```python
from build123d import *

# Parameters (mm, degrees)
SKETCH1_W           = 127
SKETCH1_H           = 266.7
BOSS_EXTRUDE1_DEPTH = 25.4
SHELL1_T            = -3.175
SKETCH2_R           = 9.525
SKETCH2_R_2         = 3.175
BOSS_EXTRUDE2_DEPTH = 3.175
BOSS_EXTRUDE3_DEPTH = 38.1


with BuildPart() as part:
    # Sketch1 → Boss-Extrude1 (new, symmetric)
    with BuildSketch(Plane.XY):
        Rectangle(SKETCH1_W, SKETCH1_H)
    extrude(amount=BOSS_EXTRUDE1_DEPTH, both=True)

    # Shell1
    shell1_openings = [part.faces().sort_by_distance(p)[0] for p in [
        (0, 0, 25.4),
    ]]
    offset(amount=SHELL1_T, openings=shell1_openings, kind=Kind.INTERSECTION)

    # Sketch2 → Boss-Extrude2 (add)
    with BuildSketch(Plane.ZY.offset(63.5)):
        with BuildLine():
            Line((50.8, 130.175), (25.4, 130.175))
            Line((25.4, 130.175), (25.4, 53.975))
            Line((25.4, 53.975), (44.45, 53.975))
            ThreePointArc((44.45, 53.975), (55.181439518, 59.883372369), (55.927786008, 72.11103057))
            ThreePointArc((55.927786008, 72.11103057), (54.690903616, 84.99461885), (61.97223251, 95.695038213))
            ThreePointArc((61.97223251, 95.695038213), (68.922407015, 116.99704087), (50.8, 130.175))
        make_face()
        with Locations(Location((50.8, 111.125, 0), (0, 0, 270))):
            Circle(SKETCH2_R, mode=Mode.SUBTRACT)
        with Locations(Location((44.45, 66.675, 0), (0, 0, 270))):
            Circle(SKETCH2_R_2, mode=Mode.SUBTRACT)
    boss_extrude2 = extrude(amount=-BOSS_EXTRUDE2_DEPTH)

    # Sketch3 → Boss-Extrude3 (add)
    with BuildSketch(Plane(origin=(0, 133.35, 0), x_dir=(1, 0, 0), z_dir=(0, 1, 0))):
        with BuildLine():
            Line((63.5, -25.4), (-63.5, -25.4))
            Line((-63.5, -25.4), (-63.5, 38.1))
            Line((-63.5, 38.1), (25.4, 38.1))
            ThreePointArc((25.4, 38.1), (52.340768363, 26.940768363), (63.5, 0))
            Line((63.5, 0), (63.5, -25.4))
        make_face()
    extrude(amount=BOSS_EXTRUDE3_DEPTH)

    # Mirror1: Boss-Extrude2 across plane
    add(boss_extrude2.mirror(Plane.ZX))


solid = part.part
```
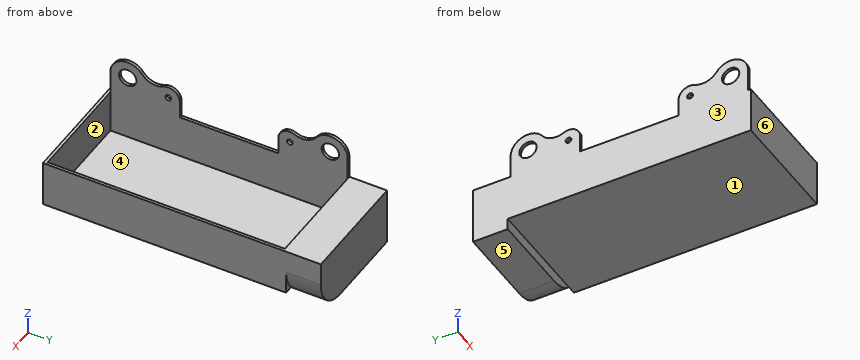
For this review, take the finished solid that the model builds, in its own axes (mm). Face numbers are marked on the shaded views. A direction names the side the tool comes from. Give positions to 0.01 mm unless a question says otherwise; leave off trailing zeros. Loops run counter-clockwise (first coordinate to the right, second up) from the corner with the lowest first, then second, coordinate; pieces in that order, holes last. Notation, with made-up numbers: M 21,-1 L 74,-1 A28 cw 74,29 Z; hole C 84.5,59 d7. An arc over 180 degrees is marked long. One line per item, written item: value. Start each with the question number.
Q1. Add section C-C (y = 139). Give the boundary of the cut face in (x, z).
Q2. For L1, parallel to X at y = -67, z = -5.5 (3 decimals); L2, parallel to Y at x = 24.5, z = -1.5 (3 decimals); L3, parallel to Z at x = 23.5, y = 33 (3 decimals), list the stretches that pass through material, from the lowest coordinate up.
Q3. Add section B-B (x = -51.5). Give the boundary of the cut face in (y, z) (3 decimals), and give its area (3 significant figures).
Q4. Add section A-A (y = 38). Give the boundary of the cut face in (x, z) (3 decimals), and give its area (3 significant figures).
Q5. Add section D-D (x = 39.5). Give the boundary of the cut face in (y, z) (3 decimals).
Q6. Draft analysis for pull direction Y (two halves, no side actions). For the marked faces 4, 5 and 6, state which applies: released by +Y, released by -Y, zero draft, split by the parting line, or undercut.
Q7. Machinability: for the marked faces 1, 2 and 3, which of the approach directions +Z, -Z, +X, -X, +Y, -Y give a long, thin tool a straight path to every point of the face, cutting with its end or side? Answer none if there is none.
Q8. Clearance check with flat-ended pins moving along their axes: pin 1 Ø2 at (x, y) = (27, 69) entering from +Z (3 decimals); pin 2 Ø8 at (x, y) = (22.5, 102) entering from -Z; pin 3 Ø1.6 at (x, z) = (-61.5, 35.5) entering from -Y (3 decimals). State where each tip first meets the part, or that it passes through.
Reply:
1. outline: M -63.5,-38.1 L 25.4,-38.1 A38.1 ccw 63.5,0 L 63.5,25.4 L -63.5,25.4 Z
2. L1: -63.5 to -60.325, 60.325 to 63.5
2. L2: -133.35 to -130.175, 130.175 to 171.45
2. L3: -25.4 to -22.225
3. outline: M -133.35,-25.4 L 133.35,-25.4 L 133.35,-38.1 L 171.45,-38.1 L 171.45,25.4 L 130.175,25.4 L 130.175,-22.225 L -130.175,-22.225 L -130.175,25.4 L -133.35,25.4 Z
3. area: 3,570 mm²
4. outline: M -63.5,-25.4 L 63.5,-25.4 L 63.5,25.4 L 60.325,25.4 L 60.325,-22.225 L -60.325,-22.225 L -60.325,25.4 L -63.5,25.4 Z
4. area: 706 mm²
5. outline: M -133.35,-25.4 L 133.35,-25.4 L 133.35,-35.395 L 171.45,-35.395 L 171.45,25.4 L 130.175,25.4 L 130.175,-22.225 L -130.175,-22.225 L -130.175,25.4 L -133.35,25.4 Z
6. face 4: undercut
6. face 5: zero draft
6. face 6: released by -Y
7. face 1: -Z, +X, -X, -Y
7. face 2: +Z
7. face 3: +Z, -Z, -X, +Y, -Y
8. pin 1: z = -22.225
8. pin 2: z = -25.4
8. pin 3: y = -130.175
